Study the drawing (mm; zero at the part's minimum x, y, z) and answer. A direction names the side the tool comes from. Coordinates: 2 decimals unless noted, no trailing zeros. Loops run counter-clockwise (first coordinate to the right, second up) from the corner with the lowest first, then second, coordinate; pieces in that order, holes last.
Q1. Section B-B (y = 19.05) is taken. Give the vertices of the cut face in (x, z) (3 decimals).
Q2. Section D-D (y = 7.5) is taken. Give the vertices of the cut face in (x, z) (3 decimals), then the cut area to 3 significant figures.
Q3. A flat-ended cylindrical pin translates along its axis: P1, Ø10, axis at y = 18.5, z = 113.5, coming from the -X side (3 decimals). Find the tip coordinate at first contact, or state that the pin passes through.
Q4. Section C-C (x = 27) is taken. Give the vertices of the cut face in (y, z) (3 decimals), then the cut area to 3 significant figures.
Q5. Straight lines are drawn through the part: line 1 (Z direction, x = 5, y = 33.5) (3 decimals); line 2 (X direction, y = 19, z = 2); line 3 (Y direction, x = 38.1, z = 1.45). For each, find the intervals that lie inside material, in ascending order.
Q6. Which of the six approach directions +Z, -Z, +X, -X, +Y, -Y give full straight-line access (tool end or side, diameter ignored) to the marked faces 1 and 2?
Q7. Section A-A (x = 38.1) is taken. Give the vertices of the cut face in (y, z) (3 decimals).
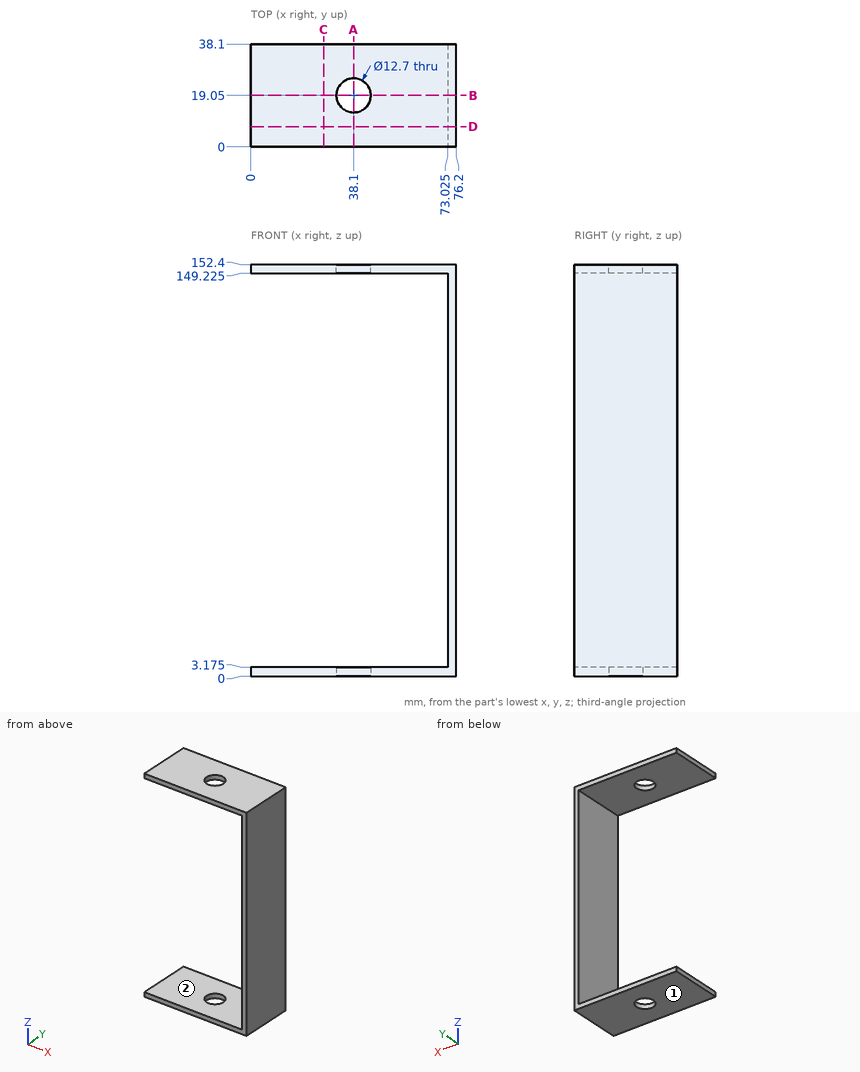
Numbers:
1. outline: (0, 0) - (31.75, 0) - (31.75, 3.175) - (0, 3.175) - close; (0, 149.225) - (31.75, 149.225) - (31.75, 152.4) - (0, 152.4) - close; (44.45, 0) - (76.2, 0) - (76.2, 152.4) - (44.45, 152.4) - (44.45, 149.225) - (73.025, 149.225) - (73.025, 3.175) - (44.45, 3.175) - close
2. outline: (0, 0) - (76.2, 0) - (76.2, 152.4) - (0, 152.4) - (0, 149.225) - (73.025, 149.225) - (73.025, 3.175) - (0, 3.175) - close
2. area: 948 mm2
3. P1: stops at x = 73.025
4. outline: (0, 0) - (38.1, 0) - (38.1, 3.175) - (0, 3.175) - close; (0, 149.225) - (38.1, 149.225) - (38.1, 152.4) - (0, 152.4) - close
4. area: 242 mm2
5. line 1: z = 0 to 3.175, 149.225 to 152.4
5. line 2: x = 0 to 31.75, 44.45 to 76.2
5. line 3: y = 0 to 12.7, 25.4 to 38.1
6. face 1: -Z, +X, -X, +Y, -Y
6. face 2: -X, +Y, -Y
7. outline: (0, 0) - (12.7, 0) - (12.7, 3.175) - (0, 3.175) - close; (0, 149.225) - (12.7, 149.225) - (12.7, 152.4) - (0, 152.4) - close; (25.4, 0) - (38.1, 0) - (38.1, 3.175) - (25.4, 3.175) - close; (25.4, 149.225) - (38.1, 149.225) - (38.1, 152.4) - (25.4, 152.4) - close
